```python
from build123d import *

# Parameters (mm, degrees)
F1_DEPTH = 300


with BuildPart() as f1:
    # F0 (on Right) → F1 (new body)
    with BuildSketch(Plane.YZ):
        with BuildLine():
            ThreePointArc((0, 0.5), (3.946913, 0.121552), (7.75, -1))
            Line((7.75, -1), (7.75, -0.5))
            ThreePointArc((7.75, -0.5), (3.946913, 0.621552), (0, 1))
            Line((0, 1), (0, 0.5))
        make_face()
        with BuildLine():
            ThreePointArc((-7.75, -1), (-3.946913, 0.121552), (0, 0.5))
            Line((0, 0.5), (0, 1))
            ThreePointArc((0, 1), (-3.946913, 0.621552), (-7.75, -0.5))
            Line((-7.75, -0.5), (-7.75, -1))
        make_face()
    extrude(amount=F1_DEPTH)


solid = f1.part
```
Verification items for the finished model (mm, model axes). Coordinates: 2 decimals unless noted, no trailing zeros. Loops run counter-clockwise (first coordinate to the right, second up) from the corner with the lowest first, then second, coordinate; pieces in that order, holes last. Notation, with made-up numbers: (33, 77.25) -> (92, 77.25) arc R16 cw to (92, 91.25) -> close; hole circle Ø9 at (56, 28). An arc over 180 degrees is marked (long way). Answer in a Markdown table with one row per item. Add a question column.
1. Material ranges on probe 1 along Z at (x, y) = (243.5, 0.5); probe 2 along Z at (x, y) = (228, 1.5), recorded low to high. Write a range as [from, to].
2. Section check A-A, the plane x = 135. Enter the section's corners in (y, z), then the cut area to 3 significant figures.
3. Depth check by flat-ended pin: P1, Ø5, axis at x = 121, y = -5, coming from the -Z side; P2, Ø1, axis at x = 237, y = 0, coming from the -Z side. Enter the tip coordinate at first touch or a pass-through.
4. Section check B-B, the plane y = 3. Enter the section's corners in (x, z).
Derived:
| question | item | result |
|---|---|---|
| 1 | probe 1 | z = [0.49, 0.99] |
| 1 | probe 2 | z = [0.45, 0.95] |
| 2 | outline | (-7.75, -1) arc R20.77 cw to (0, 0.5) arc R20.77 cw to (7.75, -1) -> (7.75, -0.5) arc R20.77 ccw to (0, 1) arc R20.77 ccw to (-7.75, -0.5) -> close |
| 2 | area | 7.75 mm² |
| 3 | P1 | stops at z = -0.9 |
| 3 | P2 | stops at z = 0.49 |
| 4 | outline | (0, 0.28) -> (300, 0.28) -> (300, 0.78) -> (0, 0.78) -> close |
